Work out the finished part from the listing and answer in its coordinate system (mm). Face numbers are marked on the shaded views. A direction names the side the tool comes from. Coordinates: 2 decimals unless noted, no trailing zeros. Order: outer loops, then holes, each group sorted by start corner. A loop starts at its lowest first (then second) coordinate and runs counter-clockwise, first axis right, second up.
1. Flat-ended cylindrical pins translate along their axes: pin 1 Ø3 at (y, z) = (0, -5) entering from -X (3 decimals); pin 2 Ø1.5 at (x, z) = (-1, 1.5) entering from -Y; pin 3 Ø1 at (x, z) = (2, -6.5) entering from -Y. Find the tip coordinate at first contact, or state that the pin passes through.
2. Find the intervals of material crossed by probe 1 along Z at (x, y) = (1.5, 0.5); probe 2 along X at (y, z) = (1.5, 10); probe 3 along Z at (x, y) = (-1.5, 4.75), in increasing order.
3. A tool of negligible diameter and unlimited length cuts with its end or side. For the marked faces 1 and 2, from which of +Z, -Z, +X, -X, +Y, -Y can it reach the whole face along a straight path? Write none if from no direction.
4. The part is cut by section A-A, the plane z = 2.5. Give the vertices of the cut face in (x, y) (3 decimals).
5. Determine the mould class of the marked faces 3, 4 and 5 for opening direction X: +X half, -X half, draft (parallel to the pull), parting line (faces both ways), or undercut.
```python
from build123d import *

# Parameters (mm, degrees)
CUT_EXTRUDE1_DEPTH = 1.84404
FILLET1_R          = 0.16764


with BuildPart() as part:
    # Sketch3 → Revolve1 (revolve)
    with BuildSketch(Plane(origin=(0, 0, 0), x_dir=(0, 0, -1), z_dir=(1, 0, 0)), mode=Mode.PRIVATE) as revolve1_sk:
        with BuildLine():
            Line((-11.2014, 0), (-11.2014, 2.778125))
            ThreePointArc((-11.2014, 2.778125), (-10.007024687, 4.401074199), (-8.35152, 5.5499))
            Line((-8.35152, 5.5499), (-7.8486, 5.461221635))
            Line((-7.8486, 5.461221635), (-7.8486, 3.175))
            Line((-7.8486, 3.175), (10.2489, 3.175))
            Line((10.2489, 3.175), (11.2014, 2.2225))
            Line((11.2014, 2.2225), (11.2014, 0))
            Line((11.2014, 0), (-11.2014, 0))
        make_face()
    revolve(revolve1_sk.sketch.rotate(Axis((0, 0, 11.2014), (0, 0, -1)), 90), axis=Axis((0, 0, 11.2014), (0, 0, -1)))

    # Sketch4 → Cut-Extrude1 (cut)
    with BuildSketch(Plane.XY.offset(11.2014)):
        Polygon((-1.984375, -1.14567944), (0, -2.291358881), (1.984375, -1.14567944), (1.984375, 1.14567944), (0, 2.291358881), (-1.984375, 1.14567944), align=None)
    extrude(amount=-CUT_EXTRUDE1_DEPTH, mode=Mode.SUBTRACT)

    # Cut-Extrude2 cone 1 section (through the dimple's axis) → Cut-Extrude2 (revolve, cut)
    with BuildSketch(Plane(origin=(0, 0, 11.2014), x_dir=(0, -1, 0), z_dir=(1, 0, 0))):
        Polygon((0, 0), (2.291358881, 0), (0, 1.322916667), align=None)
    revolve(axis=Axis((0, 0, 11.2014), (0, 0, -1)), mode=Mode.SUBTRACT)

    # Fillet1
    fillet1_edges = [part.edges().sort_by_distance(p)[0] for p in [
        (-5.461221635, 0, 7.8486),
        (-5.5499, 0, 8.35152),
    ]]
    fillet(fillet1_edges, radius=FILLET1_R)


solid = part.part
```
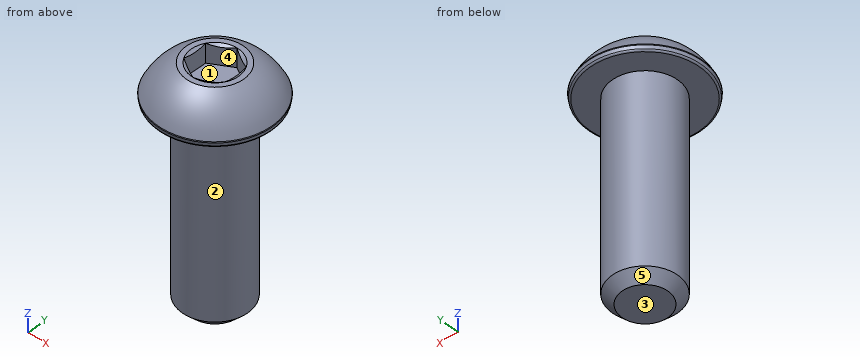
Geometry says:
1. pin 1: stops at x = -3.175
1. pin 2: stops at y = -3.17
1. pin 3: stops at y = -2.8
2. probe 1: z = -11.2 to 9.36
2. probe 2: x = -4.14 to -1.37, 1.37 to 4.14
2. probe 3: z = 7.85 to 9.32
3. face 1: +Z
3. face 2: -Z
4. outline: circle Ø6.35 at (0, 0)
5. face 3: draft
5. face 4: undercut
5. face 5: parting line
